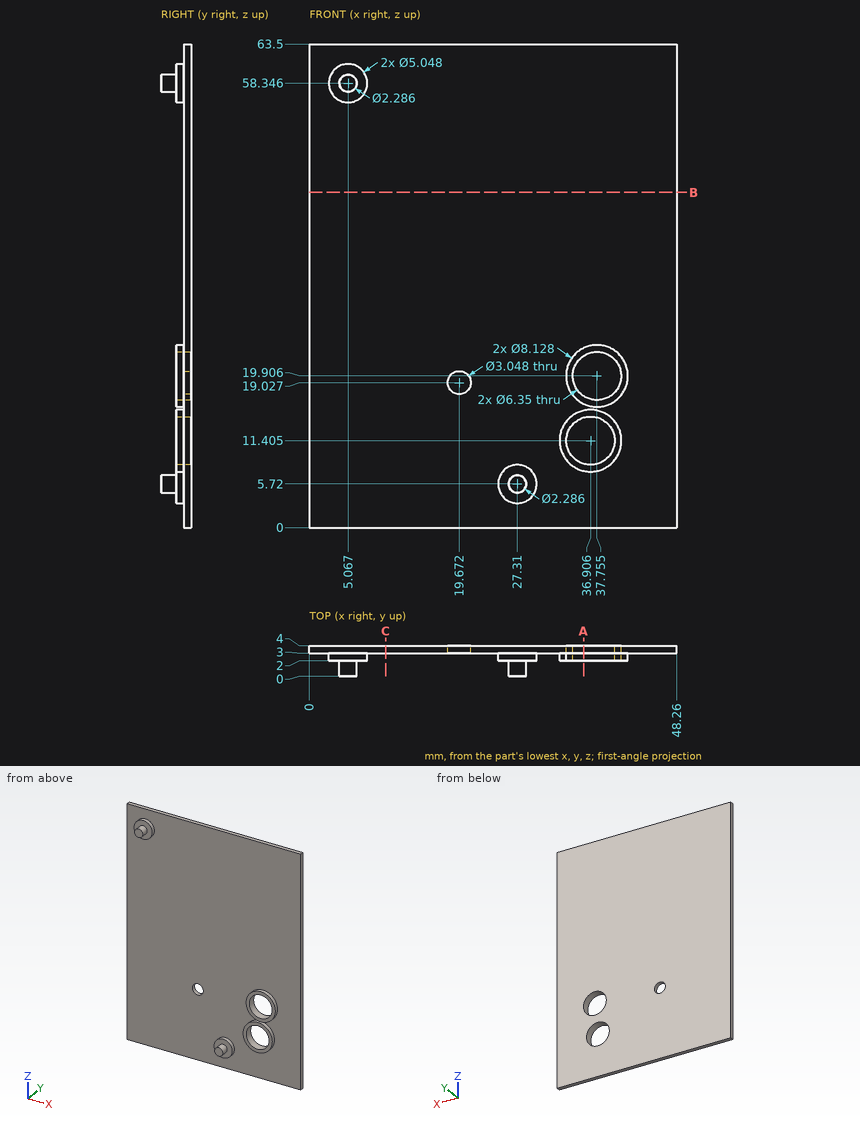
For this review, use the dimensioned drawing (mm, ordinates from the lowest corner) and the shaded views. Coordinates: 2 decimals unless noted, no trailing zeros. Write each loop counter-clockwise with the first axis right and the second up, starting at its lowest first coordinate (ties: lowest second). Pieces come first, ordered by that corner, then holes. Notation, with made-up numbers: (-21.5, -11) -> (-0.5, -11) arc R30 ccw to (-0.5, 23) -> close; hole circle Ø7 at (48.5, 76). An arc over 180 degrees is marked (long way). Put each result on its own line as item: value.
Q1. Wall thickness on L1, parallel to Y at x = 11, z = 49; L2, parallel to Z at x = 27.5, y = 1.85; L3, parallel to X at y = 2.45, z = 12 (1 decimal): over which ranges is each line inside the solid? List them lowest first.
From the geometry:
L1: y = 3 to 4
L2: z = 4.59 to 6.85
L3: x = 32.9 to 33.8, 40 to 40.9
Q2. Clearance check with flat-ended pins moving along their axes: pin 1 Ø5 at (x, z) = (16.5, 36) entering from -Y; pin 2 Ø1 at (y, z) = (2, 11) entering from +X. State where each tip first meets the part, or that it passes through.
From the geometry:
pin 1: stops at y = 3
pin 2: stops at x = 40.97
Q3. Take a section at C-C, the plane x = 10. State the section outline as (y, z) points.
From the geometry:
outline: (3, 0) -> (4, 0) -> (4, 63.5) -> (3, 63.5) -> close
Q4. Take a section at B-B, the plane z = 44. State the section outline as (x, y) points.
From the geometry:
outline: (0, 3) -> (48.26, 3) -> (48.26, 4) -> (0, 4) -> close
Q5. Take a section at A-A, the plane x = 36. State the section outline as (y, z) points.
From the geometry:
outline: (2, 7.44) -> (3, 7.44) -> (3, 0) -> (4, 0) -> (4, 8.36) -> (2, 8.36) -> close; (2, 14.45) -> (4, 14.45) -> (4, 17.26) -> (2, 17.26) -> (2, 16.24) -> (3, 16.24) -> (3, 15.37) -> (2, 15.37) -> close; (2, 22.55) -> (4, 22.55) -> (4, 63.5) -> (3, 63.5) -> (3, 23.57) -> (2, 23.57) -> close
